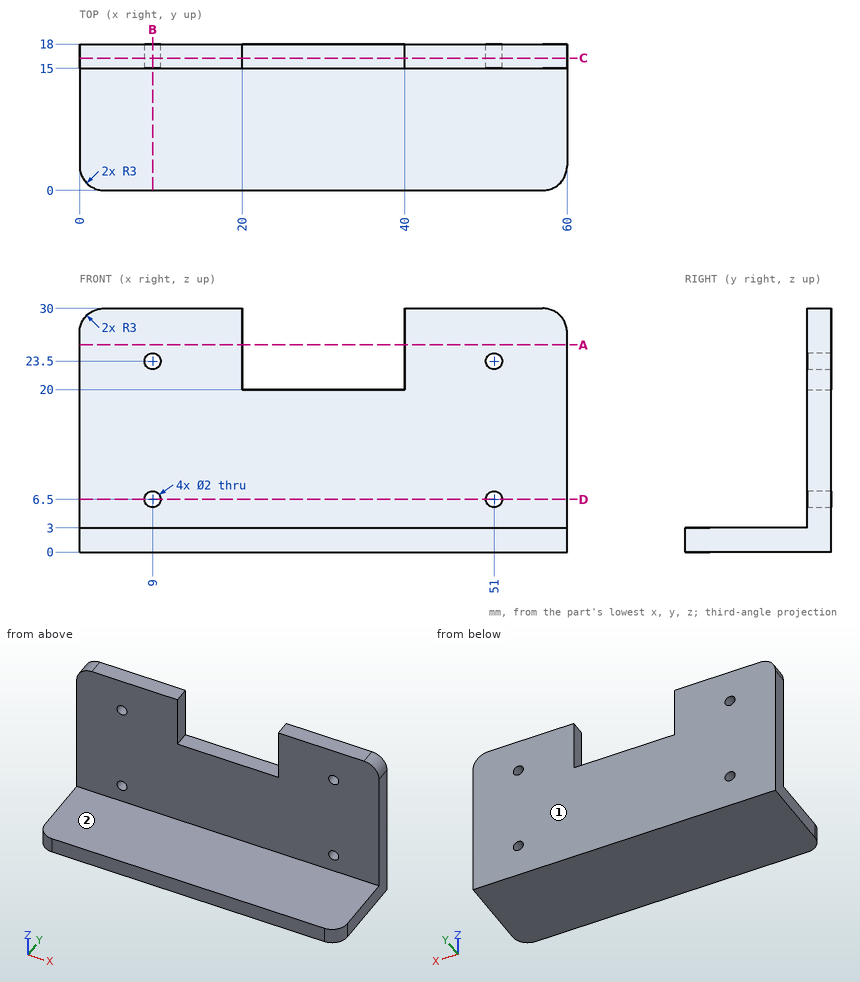
Source: three-view drawing plus pictorial views. Frame: mm from the lowest corner of the part. A direction names the side the tool comes from. Coordinates: 2 decimals unless noted, no trailing zeros. Loops run counter-clockwise (first coordinate to the right, second up) from the corner with the lowest first, then second, coordinate; pieces in that order, holes last. Notation, with made-up numbers: (-9.5, 62) -> (-5.5, 62) arc R28 cw to (-5.5, 85) -> close; hole circle Ø4 at (30.25, 81). An arc over 180 degrees is marked (long way). Write each question's results on one line, items separated by ' | '. Start each with the question number.
Q1. Pin query (flat end, axial travel): pin 1 (4 mm diameter, centred on x = 37, y = 9.5, fed in from +Z); pin 2 (10 mm diameter, centred on x = 41.5, z = 9.5, fed in from -Y); pin 3 (3.5 mm diameter, centred on x = 33.5, y = 16.5, fed in from +Z). Return the tip coordinate at first contact, or that it passes through.
Q2. Reachability of the marked faces 1 and 2 from +Z, -Z, +X, -X, +Y, -Y: full face, straight path, thin tool, end or side. Return the list, or none.
Q3. Section D-D, the plane z = 6.5. Return the cut outline in (x, y).
Q4. Ray query, line 1 (X direction, y = 15.8, z = 6.5); line 2 (Z direction, x = 51, y = 16.7); line 3 (X direction, y = 16.4, z = 23.5). Return the intervals inside material, ascending. Write a range as from..to.
Q5. Section A-A, the plane z = 25.5. Return the cut outline in (x, y).
Q6. Section C-C, the plane y = 16.25. Return the cut outline in (x, z), plus the area to 3 significant figures.
Q7. Section B-B, the plane x = 9. Return the cut outline in (y, z), plus the area to 3 significant figures.
Found:
1) pin 1: z = 3 | pin 2: y = 15 | pin 3: z = 20
2) face 1: +Z, -Z, +X, -X, +Y | face 2: +Z, +X, -X, -Y
3) outline: (0, 15) -> (8, 15) -> (8, 18) -> (0, 18) -> close; (10, 15) -> (50, 15) -> (50, 18) -> (10, 18) -> close; (52, 15) -> (60, 15) -> (60, 18) -> (52, 18) -> close
4) line 1: 0..8, 10..50, 52..60 | line 2: 0..5.5, 7.5..22.5, 24.5..30 | line 3: 0..8, 10..20, 40..50, 52..60
5) outline: (0, 15) -> (20, 15) -> (20, 18) -> (0, 18) -> close; (40, 15) -> (60, 15) -> (60, 18) -> (40, 18) -> close
6) outline: (0, 0) -> (60, 0) -> (60, 27) arc R3 ccw to (57, 30) -> (40, 30) -> (40, 20) -> (20, 20) -> (20, 30) -> (3, 30) arc R3 ccw to (0, 27) -> close; hole circle Ø2 at (9, 6.5); hole circle Ø2 at (9, 23.5); hole circle Ø2 at (51, 6.5); hole circle Ø2 at (51, 23.5) | area: 1,580 mm2
7) outline: (0, 0) -> (18, 0) -> (18, 5.5) -> (15, 5.5) -> (15, 3) -> (0, 3) -> close; (15, 7.5) -> (18, 7.5) -> (18, 22.5) -> (15, 22.5) -> close; (15, 24.5) -> (18, 24.5) -> (18, 30) -> (15, 30) -> close | area: 123 mm2
